Design review of the part built by this model. Coordinates are the model's own, in mm. A direction names the side the tool comes from. Coordinates: 2 decimals unless noted, no trailing zeros. Loops run counter-clockwise (first coordinate to the right, second up) from the corner with the lowest first, then second, coordinate; pieces in that order, holes last. Notation, with made-up numbers: (-23.75, 64) -> (-16.75, 64) arc R14 ccw to (-16.75, 76) -> close; hole circle Ø8 at (-30, 76.5). An arc over 180 degrees is marked (long way). Answer as a JSON object with one key per item and string values.
Autodesk Inventor part; units mm, degrees
ref_plane "YZ Plane" through (0, 0, 0) normal (1, 0, 0) x (0, 1, 0)
ref_plane "XZ Plane" through (0, 0, 0) normal (0, 1, 0) x (-1, 0, 0)
ref_plane "XY Plane" through (0, 0, 0) normal (0, 0, 1) x (1, 0, 0)
sketch "Sketch1" plane through (0, 0, 0) normal (0, 1, 0) x (-1, 0, 0)
  line L0 (-35, -25) -> (35, -25)
  line L1 (35, -25) -> (35, 25)
  line L2 (35, 25) -> (-35, 25)
  line L3 (-35, 25) -> (-35, -25)
  line L4 (-35, -25) -> (35, 25) construction
  line L5 (35, -25) -> (-35, 25) construction
  line L6 (25, -10) -> (25, 10)
  line L7 (-25, -10) -> (-25, 10)
  point P0 (0, 0)
  point P1 (25, 0)
  point P2 (0, 0)
  point P3 (-25, 0)
  dimension "d0" = 70
  dimension "d1" = 50
  dimension "d17" = 20
  dimension "d18" = 20
  dimension "d19" = 10
  dimension "d20" = 10
extrude "Extrusion1" add sketch "Sketch1" along normal blind 5
sketch "Sketch3" plane through (0, 0, 0) normal (0, 0, 1) x (1, 0, 0)
  circle A0 centre (0, 22.5) radius 17.5
  line L0 (-35, 5) -> (35, 5)
  circle A1 centre (0, 22.5) radius 13.75
  line L1 (17.5, 22.5) -> (17.5, 5)
  line L2 (-17.5, 22.5) -> (-17.5, 5)
  point P0 (0, 0)
  point P1 (0, 5)
  point P2 (0, 5)
  dimension "d13" = 35
  dimension "d14" = 27.5
extrude "Extrusion2" add sketch "Sketch3" along normal mid plane 20
hole "Hole2" at (-25, 0, -10) at (-25, 0, 10) at (25, 0, -10) at (25, 0, 10) direction (0, 1, 0) diameter 5.4 end through all
properties part number "base_motor"
1) Wall thickness on probe 1 along X at (y, z) = (2, -10); probe 2 along Z at (x, y) = (-25, 3.95); probe 3 along Y at (x, z) = (-1, 12): over which ranges is each line inside the solid? List them lowest first.
Completed:
{"probe 1": "-35 to -27.7, -22.3 to 22.3, 27.7 to 35", "probe 2": "-25 to -12.7, -7.3 to 7.3, 12.7 to 25", "probe 3": "0 to 5"}
2) Add section D-D, the plane y = 27. Give the boundary of the cut face in (x, z).
Completed:
{"outline": "(-16.91, -10) -> (-12.99, -10) -> (-12.99, 10) -> (-16.91, 10) -> close; (12.99, -10) -> (16.91, -10) -> (16.91, 10) -> (12.99, 10) -> close"}
3) Add section C-C, the plane x = 0. Give the boundary of the cut face in (y, z).
Completed:
{"outline": "(0, -25) -> (5, -25) -> (5, -10) -> (8.75, -10) -> (8.75, 10) -> (5, 10) -> (5, 25) -> (0, 25) -> close; (36.25, -10) -> (40, -10) -> (40, 10) -> (36.25, 10) -> close"}
4) The part is to be moulded in two halves that separate along X. For faces 6 (the cylindrical face through (22.323, 2.535, 10.351)), 7 (the flat face through (35, 2, 0)), 8 (the flat face through (0, 0, 0)), say which applies: pulls with the +X half, pulls with the -X half, needs draft (parallel to the pull), parting line crosses it, or undercut.
Completed:
{"face 6": "undercut", "face 7": "pulls with the +X half", "face 8": "needs draft"}
5) For faces 1 (the flat face through (-8, 11, 10)), 2 (the flat face through (-8, 11, -10)), 3 (the cylindrical face through (0, 40, 0)), 4 (the flat face through (-17.5, 14, 0)), 5 (the flat face through (17.5, 14, 0)), list the 3-axis set-ups (+Z, -Z, +X, -X, +Y, -Y) from which the entire face can be reached by the end or side of a thin tool; tool diameter is ignored.
Completed:
{"face 1": "+Z, +X, -X, +Y", "face 2": "-Z, +X, -X, +Y", "face 3": "+Z, -Z, +Y", "face 4": "+Z, -Z, -X, +Y", "face 5": "+Z, -Z, +X, +Y"}
6) Add section B-B, the plane y = 3. Give the boundary of the cut face in (x, z).
Completed:
{"outline": "(-35, -25) -> (35, -25) -> (35, 25) -> (-35, 25) -> close; hole circle Ø5.4 at (-25, -10); hole circle Ø5.4 at (-25, 10); hole circle Ø5.4 at (25, -10); hole circle Ø5.4 at (25, 10)"}
7) Clearance check with flat-ended pins moving along their axes: pin 1 Ø6 at (x, z) = (-23.5, -18.5) entering from +Y; pin 2 Ø4 at (x, z) = (28, 3.5) entering from -Y; pin 3 Ø12 at (x, y) = (13.5, 25) entering from +Z; pin 4 Ø4.5 at (x, z) = (-25, 10) entering from -Y. State where each tip first meets the part, or that it passes through.
Completed:
{"pin 1": "y = 5", "pin 2": "y = 0", "pin 3": "z = 10", "pin 4": "through"}
8) Add section A-A, the plane x = 25. Give the boundary of the cut face in (y, z), and give its area (3 significant figures).
Completed:
{"outline": "(0, -25) -> (5, -25) -> (5, -12.7) -> (0, -12.7) -> close; (0, -7.3) -> (5, -7.3) -> (5, 7.3) -> (0, 7.3) -> close; (0, 12.7) -> (5, 12.7) -> (5, 25) -> (0, 25) -> close", "area": "196 mm²"}
